Here's how the part is built. I have some questions about the finished solid (model axes, mm). A direction names the side the tool comes from. Give positions to 0.01 mm unless a question says otherwise; leave off trailing zeros. Write each loop counter-clockwise with the first axis right and the second up, starting at its lowest first coordinate (ties: lowest second). Pieces come first, ordered by that corner, then holes. Notation, with made-up numbers: M 55,-29.5 L 72,-29.5 A12 cw 72,-19.5 Z; hole C 30,39 d5. An arc over 180 degrees is marked long. Use one line per item in the form item = value. Start each with the question number.
from build123d import *

# Parameters (mm, degrees)
SKETCH1_W           = 80
SKETCH1_H           = 50
BOSS_EXTRUDE1_DEPTH = 3
SKETCH2_R           = 1.25
CUT_EXTRUDE1_DEPTH  = 3
SKETCH3_W           = 5
SKETCH3_H           = 4
BOSS_EXTRUDE2_DEPTH = 22
BOSS_EXTRUDE3_DEPTH = 2
FILLET1_R           = 2
SKETCH8_W           = 80
SKETCH8_H           = 8
BOSS_EXTRUDE4_DEPTH = 2
FILLET2_R           = 2
SKETCH6_R           = 1.35
CUT_EXTRUDE2_DEPTH  = 2
SKETCH12_W          = 20
SKETCH12_H          = 3
BOSS_EXTRUDE6_DEPTH = 5
SKETCH13_W          = 20
SKETCH13_H          = 1
BOSS_EXTRUDE7_DEPTH = 10
SKETCH14_R          = 1.5
CUT_EXTRUDE5_DEPTH  = 1
FILLET3_R           = 2
FILLET4_R           = 2


with BuildPart() as part:
    # Sketch1 → Boss-Extrude1 (new body)
    with BuildSketch(Plane(origin=(0, 0, 0), x_dir=(1, 0, 0), z_dir=(0, 1, 0))):
        with Locations((40, 25)):
            Rectangle(SKETCH1_W, SKETCH1_H)
    extrude(amount=BOSS_EXTRUDE1_DEPTH)

    # Sketch2 → Cut-Extrude1 (cut)
    with BuildSketch(Plane(origin=(0, 3, 0), x_dir=(1, 0, 0), z_dir=(0, 1, 0))):
        with Locations(Location((22, 43, 0), (0, 0, 270))):
            Circle(SKETCH2_R)
        with Locations(Location((58, 43, 0), (0, 0, 270))):
            Circle(SKETCH2_R)
        with Locations(Location((22, 7, 0), (0, 0, 270))):
            Circle(SKETCH2_R)
        with Locations(Location((58, 7, 0), (0, 0, 270))):
            Circle(SKETCH2_R)
    extrude(amount=-CUT_EXTRUDE1_DEPTH, mode=Mode.SUBTRACT)

    # Sketch3 → Boss-Extrude2 (add)
    with BuildSketch(Plane(origin=(0, 3, 0), x_dir=(1, 0, 0), z_dir=(0, 1, 0))):
        with Locations((22, 2)):
            Rectangle(SKETCH3_W, SKETCH3_H)
        with Locations((22, 48)):
            Rectangle(SKETCH3_W, SKETCH3_H)
        with Locations((58, 48)):
            Rectangle(SKETCH3_W, SKETCH3_H)
        with Locations((58, 2)):
            Rectangle(SKETCH3_W, SKETCH3_H)
    extrude(amount=BOSS_EXTRUDE2_DEPTH)

    # Sketch5 → Boss-Extrude3 (add)
    with BuildSketch(Plane(origin=(0, 23, 0), x_dir=(1, 0, 0), z_dir=(0, 1, 0))):
        with BuildLine():
            Line((24.5, 50), (55.5, 50))
            Line((55.5, 50), (55.5, 46))
            Line((55.5, 46), (52.660903874, 46))
            ThreePointArc((52.660903874, 46), (51.246690312, 45.414213562), (50.660903874, 44))
            Line((50.660903874, 44), (50.660903874, 6))
            ThreePointArc((50.660903874, 6), (51.246690312, 4.585786438), (52.660903874, 4))
            Line((52.660903874, 4), (55.5, 4))
            Line((55.5, 4), (55.5, 0))
            Line((55.5, 0), (24.5, 0))
            Line((24.5, 0), (24.5, 4))
            Line((24.5, 4), (24.5, 46))
            Line((24.5, 46), (24.5, 50))
        make_face()
    extrude(amount=BOSS_EXTRUDE3_DEPTH)

    # Fillet1
    fillet1_edges = [part.edges().sort_by_distance(p)[0] for p in [
        (24.5, 24, -4),
        (24.5, 24, -46),
    ]]
    fillet(fillet1_edges, radius=FILLET1_R)

    # Sketch8 → Boss-Extrude4 (add)
    with BuildSketch(Plane(origin=(0, 25, 0), x_dir=(1, 0, 0), z_dir=(0, 1, 0))):
        with Locations((40, 54)):
            Rectangle(SKETCH8_W, SKETCH8_H)
        with Locations((40, -4)):
            Rectangle(SKETCH8_W, SKETCH8_H)
    extrude(amount=-BOSS_EXTRUDE4_DEPTH)

    # Fillet2
    fillet2_edges = [part.edges().sort_by_distance(p)[0] for p in [
        (19.5, 24, 0),
        (60.5, 24, 0),
        (60.5, 24, -50),
        (19.5, 24, -50),
    ]]
    fillet(fillet2_edges, radius=FILLET2_R)

    # Sketch6 → Cut-Extrude2 (cut)
    with BuildSketch(Plane(origin=(0, 25, 0), x_dir=(1, 0, 0), z_dir=(0, 1, 0))):
        with Locations(Location((4, -2, 0), (0, 0, 270))):
            Circle(SKETCH6_R)
        with Locations(Location((4, 52, 0), (0, 0, 270))):
            Circle(SKETCH6_R)
        with Locations(Location((76, 52, 0), (0, 0, 270))):
            Circle(SKETCH6_R)
        with Locations(Location((76, -2, 0), (0, 0, 270))):
            Circle(SKETCH6_R)
    extrude(amount=-CUT_EXTRUDE2_DEPTH, mode=Mode.SUBTRACT)

    # Sketch12 → Boss-Extrude6 (add)
    with BuildSketch(Plane.XZ):
        with Locations((40, -15)):
            Rectangle(SKETCH12_W, SKETCH12_H)
        with Locations((40, -35)):
            Rectangle(SKETCH12_W, SKETCH12_H)
    extrude(amount=BOSS_EXTRUDE6_DEPTH)

    # Sketch13 → Boss-Extrude7 (add)
    with BuildSketch(Plane.XY.offset(-13.5)):
        with Locations((40, -4.5)):
            Rectangle(SKETCH13_W, SKETCH13_H)
    boss_extrude7 = extrude(amount=BOSS_EXTRUDE7_DEPTH)

    # Sketch14 → Cut-Extrude5 (cut)
    with BuildSketch(Plane(origin=(0, -4, 0), x_dir=(1, 0, 0), z_dir=(0, 1, 0))):
        with Locations(Location((40, 10, 0), (0, 0, 270))):
            Circle(SKETCH14_R)
    cut_extrude5 = extrude(amount=-CUT_EXTRUDE5_DEPTH, mode=Mode.SUBTRACT)

    # Mirror1: Boss-Extrude7, Cut-Extrude5 across plane
    add(boss_extrude7.mirror(Plane(origin=(0, 0, -25), x_dir=(1, 0, 0), z_dir=(0, 0, -1))))
    add(cut_extrude5.mirror(Plane(origin=(0, 0, -25), x_dir=(1, 0, 0), z_dir=(0, 0, -1))), mode=Mode.SUBTRACT)

    # Fillet3
    fillet3_edges = [part.edges().sort_by_distance(p)[0] for p in [
        (58, 23, -50),
        (22, 23, -50),
        (22, 23, 0),
        (58, 23, 0),
        (24.5, 23, -2),
        (24.5, 23, -48),
        (55.5, 23, -2),
        (55.5, 23, -48),
    ]]
    fillet(fillet3_edges, radius=FILLET3_R)

    # Fillet4
    fillet4_edges = [part.edges().sort_by_distance(p)[0] for p in [
        (30, 0, -35),
        (40, 0, -36.5),
        (50, 0, -35),
        (50, 0, -15),
        (40, 0, -13.5),
        (30, 0, -15),
    ]]
    fillet(fillet4_edges, radius=FILLET4_R)


solid = part.part
1) Thinking about a two-plate mould opening in Y: for faces 6 (the face through (25.1, 22.43, -48.38)), 7 (the face through (50.6, -0.57, -35.41)), 8 (the face through (24.5, 24, -25)), 9 (the face through (54.9, 22.43, -1.62)), which applies, released by +Y, released by -Y, zero draft, split by the parting line, or undercut?
2) On a 3-axis mill with a long thin cutter (end or side, diameter ignored), from which of +Z, -Z, +X, -X, +Y, -Y can I reach the whole of each face in a straight line? I mean faces 1 (the face through (39.1, -4.5, -38.8)), 2 (the face through (40, -4, -43)), 3 (the face through (40, -3, -13.5)), 4 (the face through (71, 24, -50)), 5 (the face through (23.93, 24.01, -4.6)). Say none if no direction works.
3) Suppose I cut it at C-C, the plane z = -43. List the corners of the cut face in (x, y) for me.
4) Please list where these lines run through material, in increasing order: line 1 (Y direction, x = 39.5, z = -5); line 2 (Z direction, x = 76, y = 23.9); line 3 (X direction, y = 24.5, z = 2).
5) Suppose I cut it at B-B, the plane z = -29. List the corners of the cut face in (x, y) for me.
6) Suppose I cut it at A-A, the plane x = 36.5. List the corners of the cut face in (y, z) for me, and give its area (3 significant figures).
7) Suppose I cut it at D-D, the plane x = 64.5. List the corners of the cut face in (y, z) for me, and give its area (3 significant figures).
8) Will these pins go through, and if not, where does the flat tip stop? P1, Ø10.5, axis at x = 29, y = 8.5, coming from the +Z side; P2, Ø1, axis at y = 11.5, z = -46, coming from the +X side; P3, Ø1.1, axis at x = 37.5, y = -4.5, coming from the -Z side.
Checks:
q1.face_6 = undercut
q1.face_7 = released by -Y
q1.face_8 = zero draft
q1.face_9 = undercut
q2.face_1 = -Y
q2.face_2 = -Z, +X, -X
q2.face_3 = +Z, +X, -X
q2.face_4 = +X, +Y
q2.face_5 = -X, +Y
q3.outline = M 0,0 L 20.75,0 L 20.75,3 L 0,3 Z; M 23.25,0 L 56.75,0 L 56.75,3 L 23.25,3 Z; M 24.5,23 L 50.66,23 L 50.66,25 L 24.5,25 Z; M 30,-5 L 50,-5 L 50,-4 L 30,-4 Z; M 59.25,0 L 80,0 L 80,3 L 59.25,3 Z
q4.line_1 = -5 to -4, 0 to 3, 23 to 25
q4.line_2 = -58 to -53.35, -50.65 to -50, 0 to 0.65, 3.35 to 8
q4.line_3 = 0 to 2.65, 5.35 to 74.65, 77.35 to 80
q5.outline = M 0,0 L 80,0 L 80,3 L 0,3 Z; M 24.5,23 L 50.66,23 L 50.66,25 L 24.5,25 Z
q6.outline = M -5,-46.5 L -4,-46.5 L -4,-36.5 L -2,-36.5 A2 cw 0,-38.5 L 0,-50 L 3,-50 L 3,0 L 0,0 L 0,-11.5 A2 cw -2,-13.5 L -4,-13.5 L -4,-3.5 L -5,-3.5 L -5,-16.5 L 0,-16.5 L 0,-33.5 L -5,-33.5 Z; M 23,-58 L 25,-58 L 25,8 L 23,8 Z
q6.area = 334 mm^2
q7.outline = M 0,-50 L 3,-50 L 3,0 L 0,0 Z; M 23,-58 L 25,-58 L 25,-50 L 23,-50 Z; M 23,0 L 25,0 L 25,8 L 23,8 Z
q7.area = 182 mm^2
q8.P1 = 0
q8.P2 = 60.5
q8.P3 = -46.5
